```python
from build123d import *

# Parameters (mm, degrees)
SKETCH1_W           = 120.65
SKETCH1_H           = 190.5
BOSS_EXTRUDE1_DEPTH = 6.35
CAVITY1_START       = -19.05
CAVITY1_OUTLINE_W   = 6.35
CAVITY1_OUTLINE_H   = 6.35
CAVITY1_DEPTH       = 6.35
CAVITY1_START_2     = 10.31875
CAVITY1_2_OUTLINE_W = 6.35
CAVITY1_2_OUTLINE_H = 6.35
CAVITY1_2_DEPTH     = 6.35
CAVITY1_START_3     = -6.35
CAVITY1_3_OUTLINE_W = 6.35
CAVITY1_3_OUTLINE_H = 6.35
CAVITY1_3_DEPTH     = 12.7
CAVITY1_START_4     = 19.05
CAVITY1_4_OUTLINE_W = 6.35
CAVITY1_4_OUTLINE_H = 6.35
CAVITY1_4_DEPTH     = 12.7
CAVITY1_START_5     = 44.45
CAVITY1_5_OUTLINE_W = 6.35
CAVITY1_5_OUTLINE_H = 6.35
CAVITY1_5_DEPTH     = 12.7
CAVITY1_START_6     = 69.85
CAVITY1_6_OUTLINE_W = 6.35
CAVITY1_6_OUTLINE_H = 6.35
CAVITY1_6_DEPTH     = 12.7
CAVITY1_START_7     = 95.25
CAVITY1_7_OUTLINE_W = 6.35
CAVITY1_7_OUTLINE_H = 6.35
CAVITY1_7_DEPTH     = 12.7
CAVITY1_START_8     = 120.65
CAVITY1_8_OUTLINE_W = 6.35
CAVITY1_8_OUTLINE_H = 6.35
CAVITY1_8_DEPTH     = 12.7
CAVITY1_START_9     = 146.05
CAVITY1_9_OUTLINE_W = 6.35
CAVITY1_9_OUTLINE_H = 6.35
CAVITY1_9_DEPTH     = 12.7


# Read off the part's stored shape, not the designer's step: Cavity1
with BuildPart() as part:
    # Sketch1 → Boss-Extrude1 (new body)
    with BuildSketch(Plane.XY):
        with Locations((15.875, 76.2)):
            Rectangle(SKETCH1_W, SKETCH1_H)
    extrude(amount=BOSS_EXTRUDE1_DEPTH)

    # Cavity1 outline → Cavity1 (cut)
    with BuildSketch(Plane(origin=(0, 0, 0), x_dir=(1, 0, 0), z_dir=(0, 1, 0)).offset(CAVITY1_START)):
        with Locations((66.675, -3.175)):
            Rectangle(CAVITY1_OUTLINE_W, CAVITY1_OUTLINE_H)
        with Locations((53.975, -3.175)):
            Rectangle(CAVITY1_OUTLINE_W, CAVITY1_OUTLINE_H)
        with Locations((41.275, -3.175)):
            Rectangle(CAVITY1_OUTLINE_W, CAVITY1_OUTLINE_H)
        with Locations((28.575, -3.175)):
            Rectangle(CAVITY1_OUTLINE_W, CAVITY1_OUTLINE_H)
        with Locations((15.875, -3.175)):
            Rectangle(CAVITY1_OUTLINE_W, CAVITY1_OUTLINE_H)
        with Locations((3.175, -3.175)):
            Rectangle(CAVITY1_OUTLINE_W, CAVITY1_OUTLINE_H)
        with Locations((-9.525, -3.175)):
            Rectangle(CAVITY1_OUTLINE_W, CAVITY1_OUTLINE_H)
        with Locations((-22.225, -3.175)):
            Rectangle(CAVITY1_OUTLINE_W, CAVITY1_OUTLINE_H)
        with Locations((-34.925, -3.175)):
            Rectangle(CAVITY1_OUTLINE_W, CAVITY1_OUTLINE_H)
    extrude(amount=CAVITY1_DEPTH, mode=Mode.SUBTRACT)

    # Cavity1 2 outline → Cavity1 2 (cut)
    with BuildSketch(Plane(origin=(0, 0, 0), x_dir=(1, 0, 0), z_dir=(0, 1, 0)).offset(CAVITY1_START_2)):
        with Locations((66.675, -3.175)):
            Rectangle(CAVITY1_2_OUTLINE_W, CAVITY1_2_OUTLINE_H)
        with Locations((53.975, -3.175)):
            Rectangle(CAVITY1_2_OUTLINE_W, CAVITY1_2_OUTLINE_H)
        with Locations((41.275, -3.175)):
            Rectangle(CAVITY1_2_OUTLINE_W, CAVITY1_2_OUTLINE_H)
        with Locations((28.575, -3.175)):
            Rectangle(CAVITY1_2_OUTLINE_W, CAVITY1_2_OUTLINE_H)
        with Locations((15.875, -3.175)):
            Rectangle(CAVITY1_2_OUTLINE_W, CAVITY1_2_OUTLINE_H)
        with Locations((3.175, -3.175)):
            Rectangle(CAVITY1_2_OUTLINE_W, CAVITY1_2_OUTLINE_H)
        with Locations((-9.525, -3.175)):
            Rectangle(CAVITY1_2_OUTLINE_W, CAVITY1_2_OUTLINE_H)
        with Locations((-22.225, -3.175)):
            Rectangle(CAVITY1_2_OUTLINE_W, CAVITY1_2_OUTLINE_H)
        with Locations((-34.925, -3.175)):
            Rectangle(CAVITY1_2_OUTLINE_W, CAVITY1_2_OUTLINE_H)
    extrude(amount=CAVITY1_2_DEPTH, mode=Mode.SUBTRACT)

    # Cavity1 3 outline → Cavity1 3 (cut)
    with BuildSketch(Plane(origin=(0, 0, 0), x_dir=(1, 0, 0), z_dir=(0, 1, 0)).offset(CAVITY1_START_3)):
        with Locations((73.025, -3.175)):
            Rectangle(CAVITY1_3_OUTLINE_W, CAVITY1_3_OUTLINE_H)
        with Locations((-41.275, -3.175)):
            Rectangle(CAVITY1_3_OUTLINE_W, CAVITY1_3_OUTLINE_H)
    extrude(amount=CAVITY1_3_DEPTH, mode=Mode.SUBTRACT)

    # Cavity1 4 outline → Cavity1 4 (cut)
    with BuildSketch(Plane(origin=(0, 0, 0), x_dir=(1, 0, 0), z_dir=(0, 1, 0)).offset(CAVITY1_START_4)):
        with Locations((73.025, -3.175)):
            Rectangle(CAVITY1_4_OUTLINE_W, CAVITY1_4_OUTLINE_H)
        with Locations((-41.275, -3.175)):
            Rectangle(CAVITY1_4_OUTLINE_W, CAVITY1_4_OUTLINE_H)
    extrude(amount=CAVITY1_4_DEPTH, mode=Mode.SUBTRACT)

    # Cavity1 5 outline → Cavity1 5 (cut)
    with BuildSketch(Plane(origin=(0, 0, 0), x_dir=(1, 0, 0), z_dir=(0, 1, 0)).offset(CAVITY1_START_5)):
        with Locations((73.025, -3.175)):
            Rectangle(CAVITY1_5_OUTLINE_W, CAVITY1_5_OUTLINE_H)
        with Locations((-41.275, -3.175)):
            Rectangle(CAVITY1_5_OUTLINE_W, CAVITY1_5_OUTLINE_H)
    extrude(amount=CAVITY1_5_DEPTH, mode=Mode.SUBTRACT)

    # Cavity1 6 outline → Cavity1 6 (cut)
    with BuildSketch(Plane(origin=(0, 0, 0), x_dir=(1, 0, 0), z_dir=(0, 1, 0)).offset(CAVITY1_START_6)):
        with Locations((73.025, -3.175)):
            Rectangle(CAVITY1_6_OUTLINE_W, CAVITY1_6_OUTLINE_H)
        with Locations((-41.275, -3.175)):
            Rectangle(CAVITY1_6_OUTLINE_W, CAVITY1_6_OUTLINE_H)
    extrude(amount=CAVITY1_6_DEPTH, mode=Mode.SUBTRACT)

    # Cavity1 7 outline → Cavity1 7 (cut)
    with BuildSketch(Plane(origin=(0, 0, 0), x_dir=(1, 0, 0), z_dir=(0, 1, 0)).offset(CAVITY1_START_7)):
        with Locations((73.025, -3.175)):
            Rectangle(CAVITY1_7_OUTLINE_W, CAVITY1_7_OUTLINE_H)
        with Locations((-41.275, -3.175)):
            Rectangle(CAVITY1_7_OUTLINE_W, CAVITY1_7_OUTLINE_H)
    extrude(amount=CAVITY1_7_DEPTH, mode=Mode.SUBTRACT)

    # Cavity1 8 outline → Cavity1 8 (cut)
    with BuildSketch(Plane(origin=(0, 0, 0), x_dir=(1, 0, 0), z_dir=(0, 1, 0)).offset(CAVITY1_START_8)):
        with Locations((73.025, -3.175)):
            Rectangle(CAVITY1_8_OUTLINE_W, CAVITY1_8_OUTLINE_H)
        with Locations((-41.275, -3.175)):
            Rectangle(CAVITY1_8_OUTLINE_W, CAVITY1_8_OUTLINE_H)
    extrude(amount=CAVITY1_8_DEPTH, mode=Mode.SUBTRACT)

    # Cavity1 9 outline → Cavity1 9 (cut)
    with BuildSketch(Plane(origin=(0, 0, 0), x_dir=(1, 0, 0), z_dir=(0, 1, 0)).offset(CAVITY1_START_9)):
        with Locations((73.025, -3.175)):
            Rectangle(CAVITY1_9_OUTLINE_W, CAVITY1_9_OUTLINE_H)
        with Locations((-41.275, -3.175)):
            Rectangle(CAVITY1_9_OUTLINE_W, CAVITY1_9_OUTLINE_H)
    extrude(amount=CAVITY1_9_DEPTH, mode=Mode.SUBTRACT)


solid = part.part
```
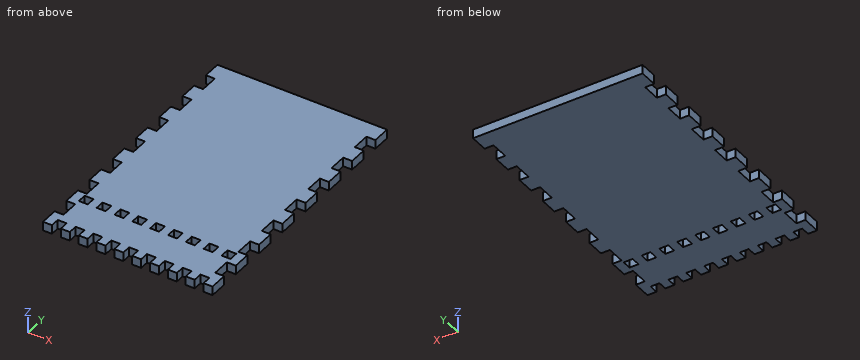
CAD build for the part. Positions are in the model's coordinates, mm. Give positions to 0.01 mm unless a question says otherwise; leave off trailing zeros. Order: outer loops, then holes, each group sorted by start corner. A loop starts at its lowest first (then second) coordinate and runs counter-clockwise, first axis right, second up.
(1) Drill centre lines: L1, parallel to Y at x = 31.5, z = 1.5; L2, parallel to X at y = 48, z = 4.75. Where is each one in solid material? Low to high.
(2) Saw through at A-A, the plane x = 17. Give the cut face in (y, z), then the cut area to 3 significant figures.
(3) Saw through at B-B, the plane z = 3. State how many separate pieces and enclosed holes the cut face has, then the cut area to 3 significant figures.
(4) Flat gauge pins, fed straight in: pin 1 (1 mm diameter, centred on x = 44, y = 33.5, fed in from -Z); pin 2 (3 mm diameter, centred on x = -35.5, z = 4, fed in from -Y); pin 3 (3 mm diameter, centred on y = 50.5, z = 2.5, fed in from -X). Where does each tip first touch, or does it go through?
(5) Saw through at C-C, the plane y = -4. Give the cut face in (x, z).
Results found:
1. L1: y = -12.7 to 10.32, 16.67 to 171.45
1. L2: x = -38.1 to 69.85
2. outline: (-12.7, 0) - (10.32, 0) - (10.32, 6.35) - (-12.7, 6.35) - close; (16.67, 0) - (171.45, 0) - (171.45, 6.35) - (16.67, 6.35) - close
2. area: 1,130 mm2
3. separate pieces: 1
3. enclosed holes: 9
3. area: 21,100 mm2
4. pin 1: stops at z = 0
4. pin 2: stops at y = -12.7
4. pin 3: stops at x = -38.1
5. outline: (-38.1, 0) - (69.85, 0) - (69.85, 6.35) - (-38.1, 6.35) - close
